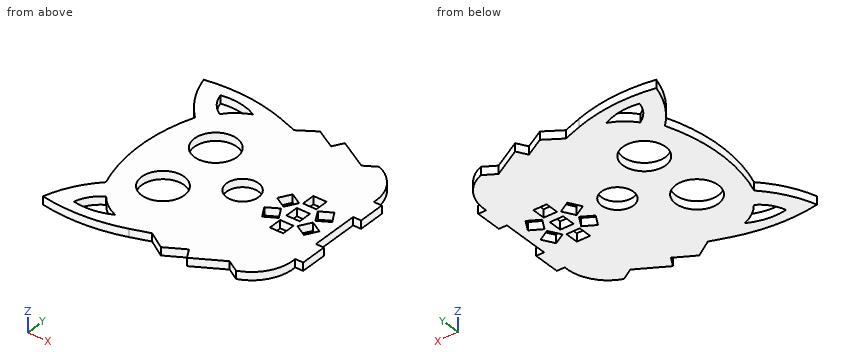
```python
from build123d import *

# Parameters (mm, degrees)
SKETCH2_R           = 8
SKETCH2_R_2         = 6
SKETCH2_W           = 5
SKETCH2_H           = 5
BOSS_EXTRUDE1_DEPTH = 3


with BuildPart() as part:
    # Sketch2 → Boss-Extrude1 (new body)
    with BuildSketch(Plane.XY):
        with BuildLine():
            Line((81.032103119, 50.181312), (81.032103119, 60.181312))
            Line((81.032103119, 60.181312), (78.032103119, 60.181312))
            ThreePointArc((78.032103119, 60.181312), (75.569321499, 69.649967364), (67.936161846, 75.770065518))
            Line((67.936161846, 75.770065518), (63.389132962, 73.023833254))
            Line((63.389132962, 73.023833254), (52.27464227, 79.356930255))
            Line((52.27464227, 79.356930255), (50.074247047, 75.495269488))
            Line((50.074247047, 75.495269488), (42.709956252, 79.691482274))
            Line((42.709956252, 79.691482274), (36.212476018, 75.495269488))
            Line((36.212476018, 75.495269488), (29.342622159, 77.861804263))
            ThreePointArc((29.342622159, 77.861804263), (14.166162437, 80.849682425), (-1.279201176, 80.017163065))
            ThreePointArc((-1.279201176, 80.017163065), (2.677054283, 70.700200378), (8.902417187, 62.718809041))
            ThreePointArc((8.902417187, 62.718809041), (5.05730693, 41.181312), (8.902417187, 19.643814959))
            ThreePointArc((8.902417187, 19.643814959), (2.677054283, 11.662423622), (-1.279201176, 2.345460935))
            ThreePointArc((-1.279201176, 2.345460935), (14.166162437, 1.512941575), (29.342622159, 4.500819737))
            Line((29.342622159, 4.500819737), (36.212476018, 6.867354512))
            Line((36.212476018, 6.867354512), (42.709956252, 2.671141726))
            Line((42.709956252, 2.671141726), (50.074247047, 6.867354512))
            Line((50.074247047, 6.867354512), (52.27464227, 3.005693745))
            Line((52.27464227, 3.005693745), (63.389132962, 9.338790746))
            Line((63.389132962, 9.338790746), (67.936161846, 6.592558482))
            ThreePointArc((67.936161846, 6.592558482), (75.569321499, 12.712656636), (78.032103119, 22.181312))
            Line((78.032103119, 22.181312), (81.032103119, 22.181312))
            Line((81.032103119, 22.181312), (81.032103119, 32.181312))
            Line((81.032103119, 32.181312), (78.032103119, 32.181312))
            Line((78.032103119, 32.181312), (78.032103119, 50.181312))
            Line((78.032103119, 50.181312), (81.032103119, 50.181312))
        make_face()
        with Locations((23.507028058, 53.931312)):
            Circle(SKETCH2_R, mode=Mode.SUBTRACT)
        with Locations((43.507028058, 41.181312)):
            Circle(SKETCH2_R_2, mode=Mode.SUBTRACT)
        with Locations((23.507028058, 28.431312)):
            Circle(SKETCH2_R, mode=Mode.SUBTRACT)
        with Locations((64.423022125, 41.181312)):
            Rectangle(SKETCH2_W, SKETCH2_H, mode=Mode.SUBTRACT)
        with Locations((64.423022125, 33.181312)):
            Rectangle(SKETCH2_W, SKETCH2_H, mode=Mode.SUBTRACT)
        Polygon((72.266288865, 48.59637551), (67.936161846, 46.09637551), (70.436161846, 41.766248491), (74.766288865, 44.266248491), align=None, mode=Mode.SUBTRACT)
        Polygon((67.936161846, 36.266248491), (72.266288865, 33.766248491), (74.766288865, 38.09637551), (70.436161846, 40.596375509), align=None, mode=Mode.SUBTRACT)
        with Locations((64.423022125, 49.181312)):
            Rectangle(SKETCH2_W, SKETCH2_H, mode=Mode.SUBTRACT)
        Polygon((56.579755385, 33.766248491), (60.909882404, 36.266248491), (58.409882404, 40.59637551), (54.079755385, 38.09637551), align=None, mode=Mode.SUBTRACT)
        Polygon((60.909882404, 46.09637551), (56.579755385, 48.596375509), (54.079755385, 44.266248491), (58.409882404, 41.766248491), align=None, mode=Mode.SUBTRACT)
        with BuildLine():
            ThreePointArc((21.611730632, 74.586477389), (14.814545044, 76.765459524), (7.678288301, 76.612049032))
            ThreePointArc((7.678288301, 76.612049032), (9.811410227, 72.018941841), (13.580912618, 68.636975763))
            ThreePointArc((13.580912618, 68.636975763), (17.183726984, 72.168659356), (21.611730632, 74.586477389))
        make_face(mode=Mode.SUBTRACT)
        with BuildLine():
            ThreePointArc((7.678288301, 5.750574968), (9.811410227, 10.343682159), (13.580912618, 13.725648237))
            ThreePointArc((13.580912618, 13.725648237), (17.183726984, 10.193964644), (21.611730632, 7.776146611))
            ThreePointArc((21.611730632, 7.776146611), (14.814545044, 5.597164476), (7.678288301, 5.750574968))
        make_face(mode=Mode.SUBTRACT)
    extrude(amount=BOSS_EXTRUDE1_DEPTH)


solid = part.part
```
Verification items for the finished model (mm, model axes). Round coordinates to 2 decimals unless told otherwise and drop trailing zeros. Order: outer loops, then holes, each group sorted by start corner. A loop starts at its lowest first (then second) coordinate and runs counter-clockwise, first axis right, second up. Notation, with made-up numbers: (13.5, -9) - (60.5, -9) arc R22 cw to (60.5, 23) - close; hole circle Ø7 at (51.25, -1.75). An arc over 180 degrees is marked (long way). Use CSV: the item, a comma, the result in double quotes.
(1) Thickness scan on probe 1 along Y at (x, z) = (73, 1.75); probe 2 along Y at (x, z) = (30.5, 1.25); probe 3 along X at (y, z) = (34.5, 0.95). Record the ranges inside material, lowest first. Write a range as from..to.
Entries:
probe 1,"9.68..35.04, 39.12..43.25, 47.33..72.68"
probe 2,"4.9..24.55, 32.32..50.05, 57.82..77.46"
probe 3,"5.42..18.29, 28.72..56.16, 57.85..61.92, 66.92..71, 72.69..78.03"
(2) Gauge pin test, flat ends, axial feed: pin 1 Ø0.9 at (x, z) = (79, 2) entering from -Y; pin 2 Ø1.5 at (y, z) = (50, 1.5) entering from -X; pin 3 Ø1.5 at (y, z) = (41.5, 1) entering from -X. Record the tip position at first contact, or that the pin passes through.
Entries:
pin 1,"y = 22.18"
pin 2,"x = 5.58"
pin 3,"x = 5.06"
(3) Section check C-C on x = 11. Record the boundary of the cut face in (y, z).
Entries:
outline,"(1.37, 0) - (5.38, 0) - (5.38, 3) - (1.37, 3) - close; (11.73, 0) - (70.64, 0) - (70.64, 3) - (11.73, 3) - close; (76.98, 0) - (80.99, 0) - (80.99, 3) - (76.98, 3) - close"
(4) Section check D-D on z = 2. State how many separate pieces and enclosed holes the cut face has, and give its area (3 significant figures).
Entries:
separate pieces,"1"
enclosed holes,"12"
area,"4,520 mm^2"
(5) Section check A-A on x = 66. Record the boundary of the cut face in (y, z).
Entries:
outline,"(7.76, 0) - (30.68, 0) - (30.68, 3) - (7.76, 3) - close; (35.68, 0) - (38.68, 0) - (38.68, 3) - (35.68, 3) - close; (43.68, 0) - (46.68, 0) - (46.68, 3) - (43.68, 3) - close; (51.68, 0) - (74.6, 0) - (74.6, 3) - (51.68, 3) - close"
(6) Section check B-B on y = 26. Record the boundary of the cut face in (x, z).
Entries:
outline,"(6.94, 0) - (15.89, 0) - (15.89, 3) - (6.94, 3) - close; (31.13, 0) - (81.03, 0) - (81.03, 3) - (31.13, 3) - close"
